Autodesk Inventor part; units mm, degrees
ref_plane "YZ Plane" through (0, 0, 0) normal (1, 0, 0) x (0, 1, 0)
ref_plane "XZ Plane" through (0, 0, 0) normal (0, 1, 0) x (-1, 0, 0)
ref_plane "XY Plane" through (0, 0, 0) normal (0, 0, 1) x (1, 0, 0)
sketch "スケッチ1" plane through (0, 0, 0) normal (0, 0, 1) x (1, 0, 0)
  line L0 (0, 0) -> (10, 0)
  line L1 (10, 0) -> (10, 275)
  line L2 (10, 275) -> (0, 275)
  line L3 (0, 275) -> (0, 0)
  dimension "d0" = 10
  dimension "d1" = 275
extrude "押し出し1" add sketch "スケッチ1" along normal blind 10
sketch "スケッチ2" plane through (10, 0, 0) normal (1, 0, 0) x (0, 0, -1)
  line L0 (0, 0) -> (-10, 0)
  line L1 (0, 275) -> (-10, 275)
  point P0 (-5, 5)
  point P1 (-5, 270)
  point P2 (-5, 0)
  point P3 (-5, 0)
  point P4 (-5, 0)
  point P5 (-5, 275)
  point P6 (-5, 0)
  point P7 (-5, 0)
  dimension "d4" = 5
  dimension "d5" = 5
hole "穴1" at (10, 5, 5) at (10, 270, 5) direction (-1, 0, 0) diameter 3.1 end through all
properties part number "SokuTate"
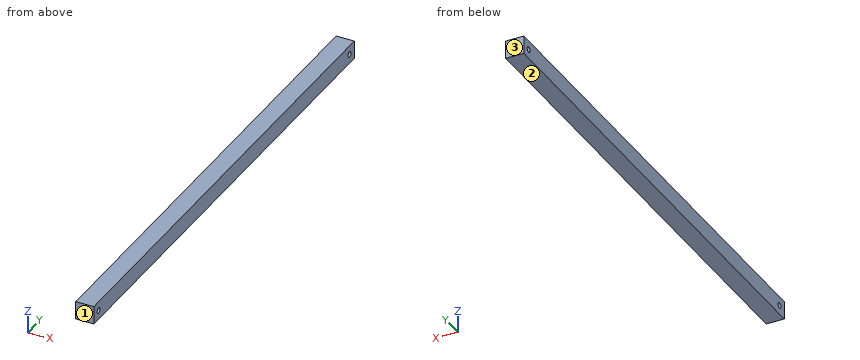
CAD build for the part. Positions are in the model's coordinates, mm. Face numbers are marked on the shaded views. Round coordinates to 2 decimals unless told otherwise and drop trailing zeros. Write each loop counter-clockwise with the first axis right and the second up, starting at its lowest first coordinate (ties: lowest second). Pieces come first, ordered by that corner, then holes.
(1) Slice it at A-A, the plane z = 5. Write the cut outline in (x, y).
(2) Mould opens along Y. For the marked faces 1, 2 and 3 say: pulls with the +Y half, pulls with the -Y half, needs draft (parallel to the pull), parting line crosses it, or undercut.
(3) Probe line 1 along Y through (x, z) = (4.25, 5); line 2 along Z through (x, y) = (4.25, 5); line 3 along Y through (x, z) = (2.5, 6). List the from-to ranges inside material, lowest first.
From the geometry:
1. outline: (0, 0) - (10, 0) - (10, 3.45) - (0, 3.45) - close; (0, 6.55) - (10, 6.55) - (10, 268.45) - (0, 268.45) - close; (0, 271.55) - (10, 271.55) - (10, 275) - (0, 275) - close
2. face 1: pulls with the -Y half
2. face 2: needs draft
2. face 3: pulls with the +Y half
3. line 1: y = 0 to 3.45, 6.55 to 268.45, 271.55 to 275
3. line 2: z = 0 to 3.45, 6.55 to 10
3. line 3: y = 0 to 3.82, 6.18 to 268.82, 271.18 to 275
